Answer from the drawing. Dimensions are ordinates in mm from the lowest x, y and z of the part. Coordinates: 2 decimals unless noted, no trailing zeros. Write each loop counter-clockwise with the first axis right and the second up, starting at its lowest first coordinate (ties: lowest second). Pieces come first, ordered by that corner, then holes.
(1) Section A-A on z = 4 is taken. Write down the section's boundary in (x, y).
(2) Section B-B on x = 10 is taken. Write down the section's boundary in (y, z).
(3) Given pin 1 (2 mm diameter, centred on y = 10, z = 4, fed in from +X), flat-ended and moving along its own axis, determine where the tip first touches the part or whether it passes through.
(4) The mould has two halves that part along X. Classify the marked faces 1, 2, 3 and 4: +X half, -X half, draft (parallel to the pull), parting line (faces both ways), or undercut.
(5) Find the intervals of material crossed by probe 1 along Z at (x, y) = (5.25, 10); probe 2 along X at (y, z) = (10, 2.5); probe 3 along Y at (x, z) = (4, 4), in increasing order.
(6) Section D-D on z = 6.25 is taken. Write down the section's boundary in (x, y), then the cut area to 3 significant figures.
(7) Section C-C on y = 10 is taken. Write down the section's boundary in (x, z), then the cut area to 3 significant figures.
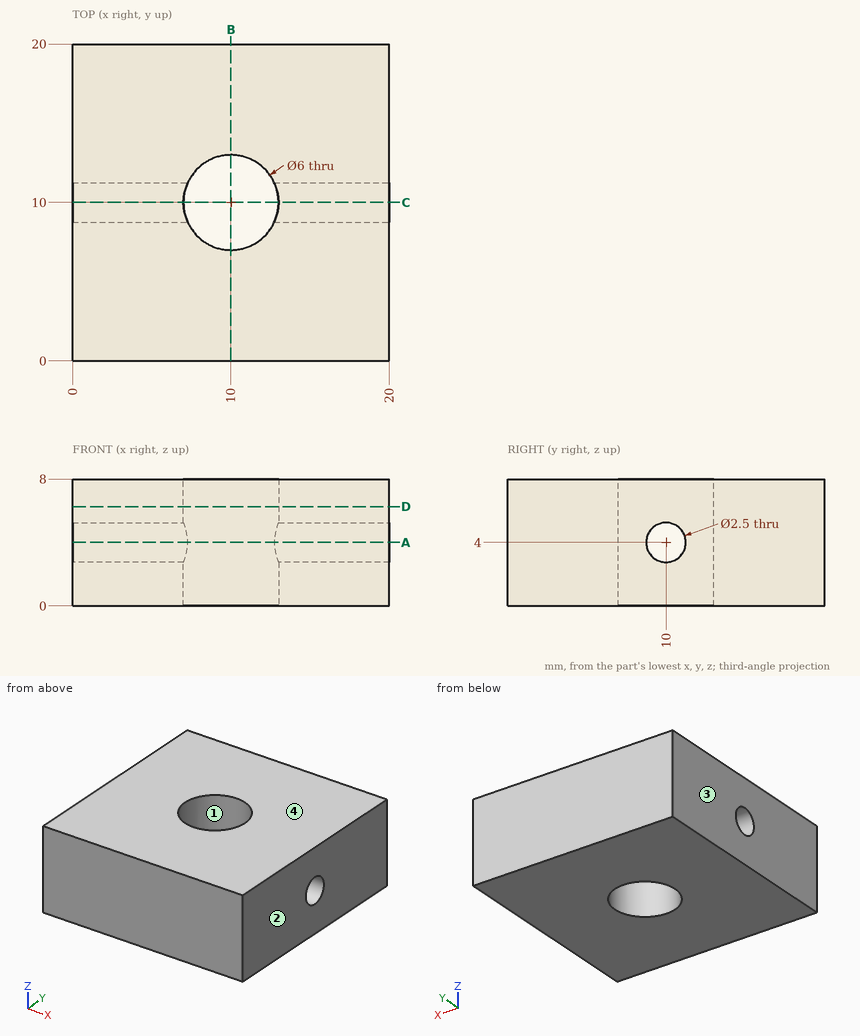
Response:
1. outline: (0, 0) - (20, 0) - (20, 8.75) - (12.73, 8.75) arc R3 cw to (7.27, 8.75) - (0, 8.75) - close; (0, 11.25) - (7.27, 11.25) arc R3 cw to (12.73, 11.25) - (20, 11.25) - (20, 20) - (0, 20) - close
2. outline: (0, 0) - (7, 0) - (7, 8) - (0, 8) - close; (13, 0) - (20, 0) - (20, 8) - (13, 8) - close
3. pin 1: passes through
4. face 1: undercut
4. face 2: +X half
4. face 3: -X half
4. face 4: draft
5. probe 1: z = 0 to 2.75, 5.25 to 8
5. probe 2: x = 0 to 7, 13 to 20
5. probe 3: y = 0 to 8.75, 11.25 to 20
6. outline: (0, 0) - (20, 0) - (20, 20) - (0, 20) - close; hole circle Ø6 at (10, 10)
6. area: 372 mm2
7. outline: (0, 0) - (7, 0) - (7, 2.75) - (0, 2.75) - close; (0, 5.25) - (7, 5.25) - (7, 8) - (0, 8) - close; (13, 0) - (20, 0) - (20, 2.75) - (13, 2.75) - close; (13, 5.25) - (20, 5.25) - (20, 8) - (13, 8) - close
7. area: 77.0 mm2
